Verification items for the finished model (mm, model axes). A direction names the side the tool comes from. Coordinates: 2 decimals unless noted, no trailing zeros. Write each loop counter-clockwise with the first axis right and the second up, starting at its lowest first coordinate (ties: lowest second). Pieces come first, ordered by that corner, then holes. Notation, with made-up numbers: (48, 18.5) -> (81, 18.5) arc R15 cw to (81, 36.5) -> close; hole circle Ø5 at (-24.5, -17). An arc over 180 degrees is marked (long way). Answer in a Markdown table with one row per item.
```python
from build123d import *

# Parameters (mm, degrees)
F0_W     = 50
F0_H     = 1.9
F1_DEPTH = 1.9
F2_DEPTH = 9.525
F3_R     = 2.5
F4_DEPTH = 1.901
F5_R     = 1.5
F6_DEPTH = 25
F7_R     = 5


with BuildPart() as f1:
    # F0 (on Front) → F1 (new body)
    with BuildSketch(Plane.XZ):
        with Locations((9.8579123784, 14.0109292623)):
            Rectangle(F0_W, F0_H)
        with BuildLine():
            ThreePointArc((-18.3860669017, 20.4335709209), (-19.169470351, 15.6888716021), (-15.1420876216, 13.0609292623))
            Line((-15.1420876216, 13.0609292623), (-15.1420876216, 14.9609292623))
            ThreePointArc((-15.1420876216, 14.9609292623), (-17.4303732633, 16.454078319), (-16.9852576671, 19.1499302047))
            Line((-16.9852576671, 19.1499302047), (-18.3860669017, 20.4335709209))
        make_face()
        Polygon((-1.496057478, 38.865271376), (-18.3860669017, 20.4335709209), (-16.9852576671, 19.1499302047), (-0.0952482434, 37.5816306598), align=None)
    extrude(amount=F1_DEPTH)

    # F2 (add, symmetric): a face of the model
    f2_faces = [f1.faces().sort_by_distance(p)[0] for p in [
        (34.2558140416, -1.9, 14.0109292623),
    ]]
    extrude(f2_faces, amount=F2_DEPTH, both=True)

    # F3 (on face) → F4 (cut, through all)
    with BuildSketch(Plane.XY.offset(14.9609292623)):
        with BuildLine():
            Line((27.8579123784, 0.6), (17.8579123784, 0.6))
            ThreePointArc((17.8579123784, 0.6), (15.3579123784, -1.9), (17.8579123784, -4.4))
            Line((17.8579123784, -4.4), (27.8579123784, -4.4))
            ThreePointArc((27.8579123784, -4.4), (30.3579123784, -1.9), (27.8579123784, 0.6))
        make_face()
        with Locations((2.8579123784, -1.9)):
            Circle(F3_R)
    extrude(amount=-F4_DEPTH, mode=Mode.SUBTRACT)

    # F5 (on face) → F6 (cut)
    with BuildSketch(Plane(origin=(-20.1719385395, 0, 18.4846879894), x_dir=(0, -1, 0), z_dir=(-0.7372680182, 0, 0.6756003769))):
        with Locations((6.925, 20.1433846083)):
            Circle(F5_R)
        with Locations((-3.125, 20.1433846083)):
            Circle(F5_R)
    extrude(amount=-F6_DEPTH, mode=Mode.SUBTRACT)

    # F7
    f7_edges = [f1.edges().sort_by_distance(p)[0] for p in [
        (-0.795653, -11.425, 38.223451),
        (-0.795653, 7.625, 38.223451),
        (34.857912, 7.625, 14.010929),
        (34.857912, -11.425, 14.010929),
    ]]
    fillet(f7_edges, radius=F7_R)


solid = f1.part
```
1. Sectioned sample at B-B, the plane y = -1.9. Record the cut outline in (x, z).
Findings below:
| item | result |
|---|---|
| outline | (-18.39, 20.43) arc R4.4 ccw to (-15.14, 13.06) -> (0.36, 13.06) -> (0.36, 14.96) -> (-15.14, 14.96) arc R2.5 cw to (-16.99, 19.15) -> (-0.1, 37.58) -> (-1.5, 38.87) -> close; (5.36, 13.06) -> (15.36, 13.06) -> (15.36, 14.96) -> (5.36, 14.96) -> close; (30.36, 13.06) -> (34.86, 13.06) -> (34.86, 14.96) -> (30.36, 14.96) -> close |
2. Release check for a two-part mould opening along X. For faces 4 (the face through (23, 0.6, 14)), 5 (the face through (0, 7.625, 14)), 6 (the face through (34.858, -2, 14)) record: released by +X, released by -X, zero draft, split by the parting line, or undercut.
Findings below:
| item | result |
|---|---|
| face 4 | undercut |
| face 5 | zero draft |
| face 6 | released by +X |
3. Access from +Z, -Z, +X, -X, +Y, -Y to the whole of each face (thin tool, end or side, straight path). Record for faces 1 (the face through (-9.82, -2.03, 29.78)), 2 (the face through (-8.658, -2.033, 28.237)), 3 (the face through (15.36, -1.85, 14.02)).
Findings below:
| item | result |
|---|---|
| face 1 | +Z, -X, +Y, -Y |
| face 2 | +X, +Y, -Y |
| face 3 | +Z, -Z |
4. Sectioned sample at D-D, the plane x = 13. Record the cut outline in (y, z) (3 decimals), and give its area (3 significant figures).
Findings below:
| item | result |
|---|---|
| outline | (-11.425, 13.061) -> (7.625, 13.061) -> (7.625, 14.961) -> (-11.425, 14.961) -> close |
| area | 36.2 mm² |
5. Go/stop test with flat-tipped pins: pin 1 (5.5 mm diameter, centred on x = 17.5, y = -3, fed in from +Z); pin 2 (1 mm diameter, centred on y = -5.5, z = 24.5, fed in from +X); pin 3 (5 mm diameter, centred on y = -4, z = 35, fed in from +X). Record where each tip stops, or that it passes through.
Findings below:
| item | result |
|---|---|
| pin 1 | stops at z = 14.96 |
| pin 2 | stops at x = -11.62 |
| pin 3 | stops at x = -0.17 |
6. Sectioned sample at C-C, the plane x = 4. Record the cut outline in (y, z) (3 decimals).
Findings below:
| item | result |
|---|---|
| outline | (-11.425, 13.061) -> (-4.124, 13.061) -> (-4.124, 14.961) -> (-11.425, 14.961) -> close; (0.324, 13.061) -> (7.625, 13.061) -> (7.625, 14.961) -> (0.324, 14.961) -> close |
7. Sectioned sample at A-A, the plane x = 24.5. Record the cut outline in (y, z) (3 decimals), and give its area (3 significant figures).
Findings below:
| item | result |
|---|---|
| outline | (-11.425, 13.061) -> (-4.4, 13.061) -> (-4.4, 14.961) -> (-11.425, 14.961) -> close; (0.6, 13.061) -> (7.625, 13.061) -> (7.625, 14.961) -> (0.6, 14.961) -> close |
| area | 26.7 mm² |
8. Material ranges on probe 1 along Z at (x, y) = (30.5, 6.5); probe 2 along Z at (x, y) = (-5.5, 6.25); probe 3 along Z at (x, y) = (-16, -7.75), recorded low to high. Write a range as from..to.
Findings below:
| item | result |
|---|---|
| probe 1 | z = 13.06..14.96 |
| probe 2 | z = 13.06..14.96, 31.68..34.5 |
| probe 3 | z = 13.15..15.11, 20.23..23.04 |
